Check sheet for the modelled part. Datum: model origin and axes. Units: mm. A direction names the side the tool comes from. Round coordinates to 2 decimals unless told otherwise and drop trailing zeros. Order: outer loops, then holes, each group sorted by start corner. A loop starts at its lowest first (then second) coordinate and runs counter-clockwise, first axis right, second up.
Q1. Mould release check, pull along Z, two halves, no side actions. Record for faces 1 (the flat face through (21, 27, -9)), 2 (the cylindrical face through (9.72, 1.61, -12.223)), 3 (the flat face through (138, 65, -19.05)), 4 (the flat face through (138, 65, 0)): +Z half, -Z half, draft (parallel to the pull), parting line (faces both ways), or undercut.
Q2. Depth check by flat-ended pin: P1, Ø6, axis at x = 22.5, z = -7, coming from the +Y side; P2, Ø5.5, axis at y = 17, z = -6, coming from the +X side (3 decimals); P3, Ø10, axis at x = 49, z = -15, coming from the +Y side. Enter the tip coordinate at first touch or a pass-through.
Q3. Cross-section at B-B on x = 151.09. Record the cut outline in (y, z) (3 decimals), then the cut area to 3 significant figures.
Q4. Scan lines: probe 1 along X at (y, z) = (25.5, -9.25) (3 decimals); probe 2 along X at (y, z) = (53.5, -5.5); probe 3 along Z at (x, y) = (151.09, 0.9) (3 decimals). Record each from-to range of solid material in increasing order.
Q5. Cross-section at A-A on y = 9. Record the cut outline in (x, z) (3 decimals), then the cut area to 3 significant figures.
Q6. Set-up check for faces 5 (the cylindrical face through (154.046, 1.61, -8.299)), 6 (the flat face through (138.09, 26, -9)), 7 (the flat face through (17.825, 28, -9)), 8 (the flat face through (141.265, 28, -9)): record each of +Z, -Z, +X, -X, +Y, -Y from which the full face is reachable in a straight line by a thin tool's end or side.
Q7. Cross-section at C-C on z = -4.5. Record the cut outline in (x, y) (3 decimals), then the cut area to 3 significant figures.
from build123d import *

# Parameters (mm, degrees)
BOSS_EXTRUDE1_DEPTH = 19.05
CUT_EXTRUDE1_REACH  = 5.175
SKETCH2_R           = 3.2
FILLET1_R           = 1


with BuildPart() as part:
    # Sketch1 → Boss-Extrude1 (new body)
    with BuildSketch(Plane.XY):
        with BuildLine():
            Line((21, 51.5), (21, 0))
            Line((21, 0), (0, 0))
            Line((0, 0), (0, 3.175))
            Line((0, 3.175), (17.825, 3.175))
            Line((17.825, 3.175), (17.825, 51.5))
            ThreePointArc((17.825, 51.5), (79.545, 113.22), (141.265, 51.5))
            Line((141.265, 51.5), (141.265, 3.175))
            Line((141.265, 3.175), (159.09, 3.175))
            Line((159.09, 3.175), (159.09, 0))
            Line((159.09, 0), (138.09, 0))
            Line((138.09, 0), (138.09, 51.5))
            ThreePointArc((138.09, 51.5), (79.545, 110.045), (21, 51.5))
        make_face()
    extrude(amount=-BOSS_EXTRUDE1_DEPTH)

    # Sketch2 → Cut-Extrude1 (cut, up to next)
    with BuildSketch(Plane(origin=(0, 3.175, 0), x_dir=(1, 0, 0), z_dir=(0, 1, 0)), mode=Mode.PRIVATE) as cut_extrude1_sk1:
        with Locations((151.09, 9.525)):
            Circle(SKETCH2_R)
    cut_extrude1_tool1 = extrude(cut_extrude1_sk1.sketch, amount=-CUT_EXTRUDE1_REACH, mode=Mode.PRIVATE) & part.part
    add(cut_extrude1_tool1.solids().sort_by_distance((151.09, 3.175, -9.525))[0], mode=Mode.SUBTRACT)
    # Sketch2 → Cut-Extrude1 (cut, up to next)
    with BuildSketch(Plane(origin=(0, 3.175, 0), x_dir=(1, 0, 0), z_dir=(0, 1, 0)), mode=Mode.PRIVATE) as cut_extrude1_sk2:
        with Locations((8, 9.525)):
            Circle(SKETCH2_R)
    cut_extrude1_tool2 = extrude(cut_extrude1_sk2.sketch, amount=-CUT_EXTRUDE1_REACH, mode=Mode.PRIVATE) & part.part
    add(cut_extrude1_tool2.solids().sort_by_distance((8, 3.175, -9.525))[0], mode=Mode.SUBTRACT)

    # Fillet1
    fillet1_edges = [part.edges().sort_by_distance(p)[0] for p in [
        (0, 1.5875, 0),
        (8.9125, 3.175, 0),
        (17.825, 27.3375, 0),
        (79.545, 113.22, 0),
        (141.265, 27.3375, 0),
        (150.1775, 3.175, 0),
        (159.09, 1.5875, 0),
        (159.09, 1.5875, -19.05),
        (21, 0, -9.525),
        (150.1775, 3.175, -19.05),
        (0, 3.175, -9.525),
        (17.825, 3.175, -9.525),
        (141.265, 3.175, -9.525),
        (159.09, 3.175, -9.525),
        (138.09, 0, -9.525),
        (141.265, 27.3375, -19.05),
        (79.545, 113.22, -19.05),
        (17.825, 27.3375, -19.05),
        (8.9125, 3.175, -19.05),
        (0, 1.5875, -19.05),
    ]]
    fillet(fillet1_edges, radius=FILLET1_R)


solid = part.part
Results found:
1. face 1: draft
1. face 2: undercut
1. face 3: -Z half
1. face 4: +Z half
2. P1: stops at y = 81.31
2. P2: stops at x = 141.265
2. P3: stops at y = 107.69
3. outline: (0, -19.05) - (2.175, -19.05) arc R1 ccw to (3.175, -18.05) - (3.175, -12.725) - (0, -12.725) - close; (0, -6.325) - (3.175, -6.325) - (3.175, -1) arc R1 ccw to (2.175, 0) - (0, 0) - close
3. area: 39.7 mm2
4. probe 1: x = 17.825 to 21, 138.09 to 141.265
4. probe 2: x = 17.86 to 21.03, 138.06 to 141.23
4. probe 3: z = -19.05 to -12.725, -6.325 to 0
5. outline: (17.825, -18.05) arc R1 ccw to (18.825, -19.05) - (21, -19.05) - (21, 0) - (18.825, 0) arc R1 ccw to (17.825, -1) - close; (138.09, -19.05) - (140.265, -19.05) arc R1 ccw to (141.265, -18.05) - (141.265, -1) arc R1 ccw to (140.265, 0) - (138.09, 0) - close
5. area: 120 mm2
6. face 5: +Y, -Y
6. face 6: +Z, -Z, -Y
6. face 7: +Z, -Z, -X, +Y
6. face 8: +Z, -Z, +X, +Y
7. outline: (0, 0) - (20, 0) arc R1 ccw to (21, 1) - (21, 51.5) arc R58.545 cw to (138.09, 51.5) - (138.09, 1) arc R1 ccw to (139.09, 0) - (159.09, 0) - (159.09, 2.175) arc R1 ccw to (158.09, 3.175) - (142.265, 3.175) arc R1 cw to (141.265, 4.175) - (141.265, 51.5) arc R61.72 ccw to (17.825, 51.5) - (17.825, 4.175) arc R1 cw to (16.825, 3.175) - (1, 3.175) arc R1 ccw to (0, 2.175) - close
7. area: 1,040 mm2
